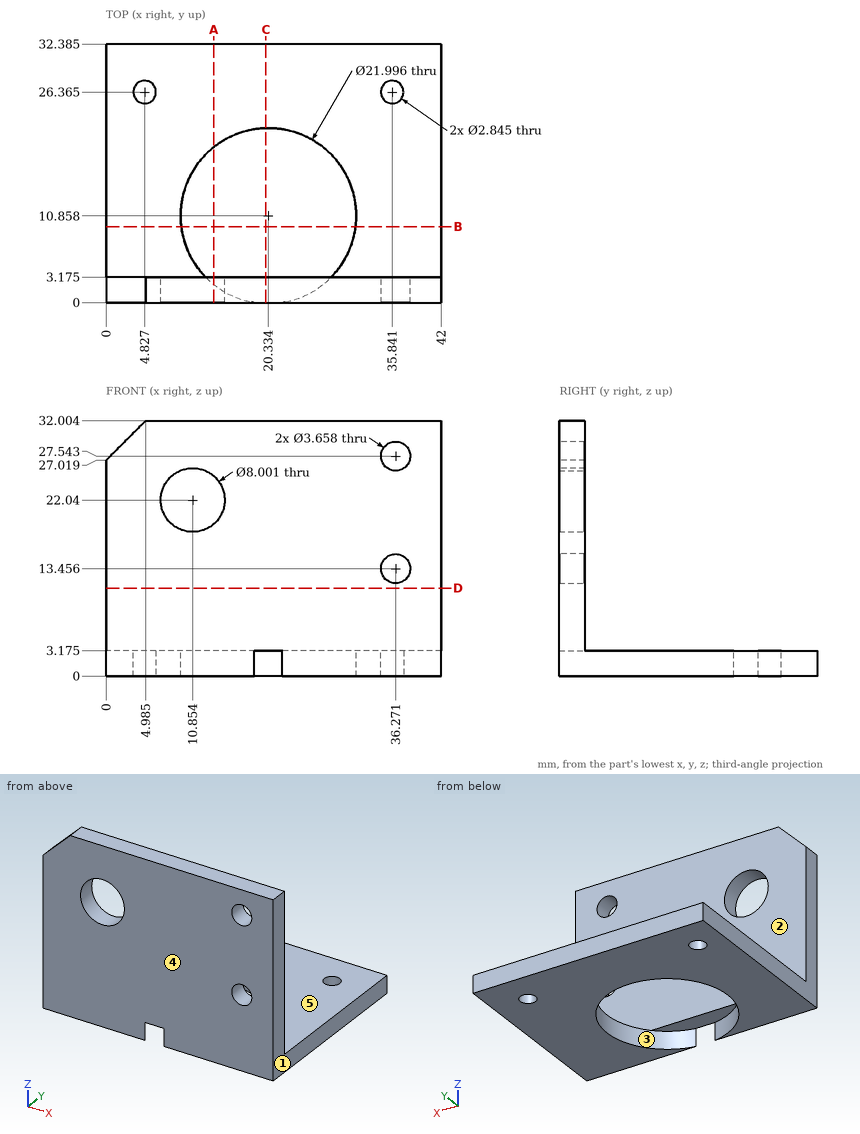
Part print with two shaded views. Sizes in mm from the minimum x, y, z corner. A direction names the side the tool comes from. Round coordinates to 2 decimals unless told otherwise and drop trailing zeros. Loops run counter-clockwise (first coordinate to the right, second up) from the corner with the lowest first, then second, coordinate; pieces in that order, holes last. Notation, with made-up numbers: (8.25, 27.25) - (26.25, 27.25) arc R21 cw to (26.25, 53.25) - close; hole circle Ø3 at (11.25, -31.5). An arc over 180 degrees is marked (long way). Put each result on its own line as item: value.
1. Slice it at D-D on z = 11. List the corners of the cut face in (x, y) (1 decimal).
Geometry check:
outline: (0, 0) - (42, 0) - (42, 3.2) - (0, 3.2) - close
2. Slice it at B-B on y = 9.5. List the corners of the cut face in (x, z) (1 decimal).
Geometry check:
outline: (0, 0) - (9.4, 0) - (9.4, 3.2) - (0, 3.2) - close; (31.2, 0) - (42, 0) - (42, 3.2) - (31.2, 3.2) - close
3. Wall check: line 1 (Y direction, x = 19, z = 24) (1 decimal). Give the ranges that are in metal, low to high.
Geometry check:
line 1: 0 to 3.2
4. Pin check, flat tips, straight feed: P1, Ø3, axis at x = 36.27, z = 13.46, coming from the -Y side; P2, Ø4, axis at x = 28.5, z = 6.5, coming from the +Y side (1 decimal); P3, Ø3.5, axis at x = 20, y = 2.5, coming from the -Z side (1 decimal); P4, Ø4, axis at x = 21.5, y = 25, coming from the +Z side (1 decimal). Stop position of each tip, or through.
Geometry check:
P1: through
P2: y = 3.2
P3: z = 3.2
P4: z = 3.2
5. Slice it at C-C on x = 20. List the corners of the cut face in (y, z) (1 decimal).
Geometry check:
outline: (0, 3.2) - (3.2, 3.2) - (3.2, 32) - (0, 32) - close; (21.9, 0) - (32.4, 0) - (32.4, 3.2) - (21.9, 3.2) - close
6. Slice it at A-A on x = 13.5. List the corners of the cut face in (y, z) (1 decimal).
Geometry check:
outline: (0, 0) - (2.2, 0) - (2.2, 3.2) - (3.2, 3.2) - (3.2, 19) - (0, 19) - close; (0, 25) - (3.2, 25) - (3.2, 32) - (0, 32) - close; (19.5, 0) - (32.4, 0) - (32.4, 3.2) - (19.5, 3.2) - close
7. 3-axis set-ups, long thin cutter, end or side, ignore diameter. For the marked faces 1 and 2: which of +Z, -Z, +X, -X, +Y, -Y reach the whole face in a straight line?
Geometry check:
face 1: +Z, -Z, +X, +Y, -Y
face 2: +Z, +X, -X, +Y
8. Two-plate mould, pull along Y, no slides. Class the marked faces 3, 4 and 5: released by +Y, released by -Y, zero draft, split by the parting line, or undercut.
Geometry check:
face 3: undercut
face 4: released by -Y
face 5: zero draft
